```python
from build123d import *

# Parameters (mm, degrees)
CYLINDER015_R     = 0.95
CYLINDER015_DEPTH = 10
CYLINDER016_R     = 0.95
CYLINDER016_DEPTH = 10
CYLINDER013_R     = 0.95
CYLINDER013_DEPTH = 10
CYLINDER014_R     = 0.95
CYLINDER014_DEPTH = 10
BOX003_W          = 10
BOX003_H          = 10
BOX003_DEPTH      = 7
PAD003_DEPTH      = 21
CYLINDER012_R     = 3
CYLINDER012_DEPTH = 10


with BuildPart() as cylinder015:
    # Cylinder015 → Cylinder015 (new body)
    with BuildSketch(Plane(origin=(9.9, 0, 0), x_dir=(1, 0, 0), z_dir=(0, 0, 1))):
        Circle(CYLINDER015_R)
    extrude(amount=CYLINDER015_DEPTH)


with BuildPart() as tornillos007:
    # Cylinder016 → Cylinder016 (new body)
    with BuildSketch(Plane.XY):
        Circle(CYLINDER016_R)
    extrude(amount=CYLINDER016_DEPTH)

    # Fusion011: union Cylinder015
    add(cylinder015.part)


with BuildPart() as tornillos007_1:
    # Fusion011 placement: moved
    add(tornillos007.part.moved(Location((5, -24.5, 22))))


with BuildPart() as cylinder013:
    # Cylinder013 → Cylinder013 (new body)
    with BuildSketch(Plane(origin=(9.9, 0, 0), x_dir=(1, 0, 0), z_dir=(0, 0, 1))):
        Circle(CYLINDER013_R)
    extrude(amount=CYLINDER013_DEPTH)


with BuildPart() as fusion012:
    # Cylinder014 → Cylinder014 (new body)
    with BuildSketch(Plane.XY):
        Circle(CYLINDER014_R)
    extrude(amount=CYLINDER014_DEPTH)

    # Fusion010: union Cylinder013
    add(cylinder013.part)


with BuildPart() as fusion012_1:
    # Fusion010 placement: moved
    add(fusion012.part.moved(Location((5, 24.5, 22))))

    # Fusion012: union Tornillos007
    add(tornillos007_1.part)


with BuildPart() as fusion012_2:
    # Fusion012 placement: moved
    add(fusion012_1.part.moved(Location((0.4, 0, 0))))


with BuildPart() as cube003:
    # Box003 → Box003 (new body)
    with BuildSketch(Plane(origin=(5, -29, 7), x_dir=(1, 0, 0), z_dir=(0, 0, 1))):
        with Locations((5, 5)):
            Rectangle(BOX003_W, BOX003_H)
    extrude(amount=BOX003_DEPTH)


with BuildPart() as holder004:
    # Sketch003 → Pad003 (new body)
    with BuildSketch(Plane.YZ):
        Polygon((-28.75, 32), (-28.75, 0), (28.75, 0), (28.75, 32), (20.75, 32), (20.75, 3.5), (-20.75, 3.5), (-20.75, 32), align=None)
    extrude(amount=PAD003_DEPTH)

    # Cut006: cut Cube003
    add(cube003.part, mode=Mode.SUBTRACT)

    # Cut007: cut Fusion012
    add(fusion012_2.part, mode=Mode.SUBTRACT)


with BuildPart() as obj1:
    # Cylinder012 → Cylinder012 (new body)
    with BuildSketch(Plane(origin=(10.5, -10.1, -7), x_dir=(1, 0, 0), z_dir=(0, 0, 1))):
        Circle(CYLINDER012_R)
    extrude(amount=CYLINDER012_DEPTH)

    # Fusion013: union Holder004
    add(holder004.part)


solid = obj1.part
```
The listing builds one solid part. Answer for the finished solid, in the listing's coordinates (mm). A direction names the side the tool comes from. Round coordinates to 2 decimals unless told otherwise and drop trailing zeros. Order: outer loops, then holes, each group sorted by start corner. A loop starts at its lowest first (then second) coordinate and runs counter-clockwise, first axis right, second up. Notation, with made-up numbers: (18, 18) - (67, 18) arc R17 cw to (67, 37) - close; hole circle Ø7 at (24.25, 24). An arc over 180 degrees is marked (long way). Put each result on its own line as item: value. Start each with the question number.
(1) Find section A-A (x = 10.5). Give the vertices of the cut face in (y, z).
(2) Find section B-B (z = 16.5). Give the vertices of the cut face in (x, y).
(3) Given P1, Ø1.5, axis at x = 15.3, y = -24.5, coming from the +Z side; P2, Ø3, axis at x = 13, y = -6, coming from the +Z side; P3, Ø5, axis at x = 2.5, y = 4.5, coming from the -Z side, each flat-ended and moving along its own axis, determine where each tip first touches the part or whether it passes through.
(4) Find section C-C (y = 24.5). Give the vertices of the cut face in (x, z).
(5) Straight lines are drawn through the part: probe 1 along Y at (x, z) = (5.4, 25); probe 2 along Y at (x, z) = (7, 18); probe 3 along X at (y, z) = (-24, 27). For each, find the intervals that lie inside material, in ascending order. Write a range as from..to.
(6) For faces 5 (the cylindrical face through (5.194, -25.427, 26.93)), 6 (the flat face through (10, 20.75, 18)), 7 (the flat face through (10, -28.75, 16)), 8 (the cylindrical face through (8.29, -8.07, -3.55)), determine the directions among +Z, -Z, +X, -X, +Y, -Y from which every point of the face is accessible in a straight line to the end or side of a thin tool.
(7) Determine the mould class of faces 1 (the flat face through (10, -25, 14)), 2 (the flat face through (10, -25, 7)), 3 (the cylindrical face through (15.094, 23.573, 26.93)), 4 (the flat face through (5, -24, 22)) for opening direction Z: released by +Z, released by -Z, zero draft, split by the parting line, or undercut.
(8) Find section D-D (x = 18.75). Give the vertices of the cut face in (y, z).
Reply:
1. outline: (-28.75, 0) - (-13.1, 0) - (-13.1, -7) - (-7.1, -7) - (-7.1, 0) - (28.75, 0) - (28.75, 32) - (20.75, 32) - (20.75, 3.5) - (-20.75, 3.5) - (-20.75, 7) - (-28.75, 7) - close; (-28.75, 14) - (-20.75, 14) - (-20.75, 32) - (-28.75, 32) - close
2. outline: (0, -28.75) - (21, -28.75) - (21, -20.75) - (0, -20.75) - close; (0, 20.75) - (21, 20.75) - (21, 28.75) - (0, 28.75) - close
3. P1: z = 22
3. P2: z = 3.5
3. P3: z = 0
4. outline: (0, 0) - (21, 0) - (21, 32) - (16.25, 32) - (16.25, 22) - (14.35, 22) - (14.35, 32) - (6.35, 32) - (6.35, 22) - (4.45, 22) - (4.45, 32) - (0, 32) - close
5. probe 1: -28.75..-25.45, -23.55..-20.75, 20.75..23.55, 25.45..28.75
5. probe 2: -28.75..-20.75, 20.75..28.75
5. probe 3: 0..4.59, 6.21..14.49, 16.11..21
6. face 5: +Z
6. face 6: +Z, +X, -X
6. face 7: +Z, -Z, +X, -X, -Y
6. face 8: -Z
7. face 1: undercut
7. face 2: undercut
7. face 3: zero draft
7. face 4: released by +Z
8. outline: (-28.75, 0) - (28.75, 0) - (28.75, 32) - (20.75, 32) - (20.75, 3.5) - (-20.75, 3.5) - (-20.75, 32) - (-28.75, 32) - close
